Here's how the part is built. I have some questions about the finished solid (model axes, mm). A direction names the side the tool comes from. Coordinates: 2 decimals unless noted, no trailing zeros. Write each loop counter-clockwise with the first axis right and the second up, starting at its lowest first coordinate (ties: lowest second). Pieces come first, ordered by that corner, then holes. Notation, with made-up numbers: M -2.5,68 L 52.5,68 A29 ccw 52.5,100 Z; hole C 3.5,58.25 d5. An arc over 180 degrees is marked long. Use a Markdown table: item, result.
```python
from build123d import *

# Parameters (mm, degrees)
SKETCH2_R               = 12.5
CUT_EXTRUDE1_DEPTH      = 62.23724357
CUT_EXTRUDE4_DEPTH      = 62.23724357
CUT_EXTRUDE4_DEPTH_BACK = 62.23724357
SKETCH5_R               = 3
BOSS_EXTRUDE1_DEPTH     = 2.5


with BuildPart() as part:
    # Sketch1 → Revolve1 (revolve)
    with BuildSketch(Plane.XY, mode=Mode.PRIVATE) as revolve1_sk:
        Polygon((-25, 0), (25, 0), (25, 25), (18, 25), (18, 19), (11, 19), (11, 17.5), (-11, 17.5), (-11, 19), (-18, 19), (-18, 25), (-25, 25), align=None)
    revolve(revolve1_sk.sketch.rotate(Axis((-25, 0, 0), (1, 0, 0)), 90), axis=Axis((-25, 0, 0), (1, 0, 0)))

    # Sketch2 → Cut-Extrude1 (cut, through all)
    with BuildSketch(Plane(origin=(25, 0, 0), x_dir=(0, 0, -1), z_dir=(1, 0, 0))):
        Circle(SKETCH2_R)
    extrude(amount=-CUT_EXTRUDE1_DEPTH, mode=Mode.SUBTRACT)

    # Sketch3 → Cut-Extrude4 (cut, two sides: drawn at the far end of the back side and taken through both)
    with BuildSketch(Plane(origin=(25, 0, 0), x_dir=(0, 0, -1), z_dir=(1, 0, 0)).offset(-CUT_EXTRUDE4_DEPTH_BACK)):
        Polygon((-146.803398875, 0), (-25, 0), (25, 0), (146.803398875, 0), (146.803398875, 243.60679775), (-146.803398875, 243.60679775), align=None)
    extrude(amount=CUT_EXTRUDE4_DEPTH + CUT_EXTRUDE4_DEPTH_BACK, mode=Mode.SUBTRACT)

    # Sketch5 → Boss-Extrude1 (add, symmetric)
    with BuildSketch(Plane(origin=(0, -17.5, 0), x_dir=(1, 0, 0), z_dir=(0, 1, 0))):
        with Locations(Location((0, 0, 0), (0, 0, 90))):
            Circle(SKETCH5_R)
    extrude(amount=BOSS_EXTRUDE1_DEPTH, both=True)


solid = part.part
```
1. I need wall thicknesses on probe 1 along X at (y, z) = (-18.75, -15); probe 2 along X at (y, z) = (-3.5, 18); probe 3 along Z at (x, y) = (-3, -1). Which ranges of each line are inside material? Lowest first, please.
Answers follow:
| item | result |
|---|---|
| probe 1 | x = -25 to -18, 18 to 25 |
| probe 2 | x = -25 to -11, 11 to 25 |
| probe 3 | z = -17.47 to -12.46, 12.46 to 17.47 |
2. Which directions (+Z, -Z, +X, -X, +Y, -Y) give clear straight access to the entire face, cutting with the end or side of a thin tool? Please do faces 1 (the face through (-11, -18, 0)), 2 (the face through (-21.549, -24.994, 0.55)), 3 (the face through (0, -20, 0)).
Answers follow:
| item | result |
|---|---|
| face 1 | -Y |
| face 2 | +X, -X, -Y |
| face 3 | +Z, -Z, -Y |
3. Will these pins go through, and if not, where does the flat tip stop? pin 1 Ø4 at (x, z) = (-2.5, -11) entering from -Y; pin 2 Ø3 at (x, z) = (0, -1.5) entering from -Y; pin 3 Ø6 at (x, y) = (-18, -19) entering from +Z; pin 4 Ø4 at (y, z) = (-22, 18.5) entering from -X.
Answers follow:
| item | result |
|---|---|
| pin 1 | stops at y = -15.01 |
| pin 2 | stops at y = -20 |
| pin 3 | stops at z = 19.21 |
| pin 4 | passes through |
4. Suppose I cut it at D-D on y = -4. Write out the boundary of the cut face in (x, z), and give its area (3 significant figures).
Answers follow:
| item | result |
|---|---|
| outline | M -25,-24.68 L -18,-24.68 L -18,-18.57 L -11,-18.57 L -11,-17.04 L 11,-17.04 L 11,-18.57 L 18,-18.57 L 18,-24.68 L 25,-24.68 L 25,-11.84 L -25,-11.84 Z; M -25,11.84 L 25,11.84 L 25,24.68 L 18,24.68 L 18,18.57 L 11,18.57 L 11,17.04 L -11,17.04 L -11,18.57 L -18,18.57 L -18,24.68 L -25,24.68 Z |
| area | 776 mm2 |
5. Suppose I cut it at A-A on y = -9. Write out the boundary of the cut face in (x, z), and give its area (3 significant figures).
Answers follow:
| item | result |
|---|---|
| outline | M -25,-23.32 L -18,-23.32 L -18,-16.73 L -11,-16.73 L -11,-15.01 L 11,-15.01 L 11,-16.73 L 18,-16.73 L 18,-23.32 L 25,-23.32 L 25,-8.67 L -25,-8.67 Z; M -25,8.67 L 25,8.67 L 25,23.32 L 18,23.32 L 18,16.73 L 11,16.73 L 11,15.01 L -11,15.01 L -11,16.73 L -18,16.73 L -18,23.32 L -25,23.32 Z |
| area | 914 mm2 |
6. We'd pull the mould along X, two halves only. Please class faces 4 (the face through (-15, -19, 0)), 5 (the face through (0.35, -12.497, 0.275)), 6 (the face through (-25, -13, 0)): +X half, -X half, draft (parallel to the pull), parting line (faces both ways), or undercut.
Answers follow:
| item | result |
|---|---|
| face 4 | undercut |
| face 5 | draft |
| face 6 | -X half |
7. Suppose I cut it at B-B on x = 0. Write out the boundary of the cut face in (y, z).
Answers follow:
| item | result |
|---|---|
| outline | M -20,-3 L -17.24,-3 A17.5 ccw 0,-17.5 L 0,-12.5 A12.5 cw 0,12.5 L 0,17.5 A17.5 ccw -17.24,3 L -20,3 Z |
8. Suppose I cut it at C-C on z = 0. Write out the boundary of the cut face in (x, y).
Answers follow:
| item | result |
|---|---|
| outline | M -25,-25 L -18,-25 L -18,-19 L -11,-19 L -11,-17.5 L -3,-17.5 L -3,-20 L 3,-20 L 3,-17.5 L 11,-17.5 L 11,-19 L 18,-19 L 18,-25 L 25,-25 L 25,-12.5 L -25,-12.5 Z |
